from build123d import *


with BuildPart() as part:
    # Sketch1 → Revolve1 (revolve)
    with BuildSketch(Plane.XY):
        with BuildLine():
            Line((0, 8), (4.7, 8))
            ThreePointArc((4.7, 8), (4.912132034, 7.912132034), (5, 7.7))
            Line((5, 7.7), (5, 3))
            Line((5, 3), (3.5, 2))
            Line((3.5, 2), (3.5, 1.5))
            Line((3.5, 1.5), (5, 0.5))
            Line((5, 0.5), (4.711324865, 0))
            Line((4.711324865, 0), (0, 0))
            Line((0, 0), (0, 8))
        make_face()
    revolve(axis=Axis((0, 0, 0), (0, 1, 0)))

    # Sketch2 → Cut-Revolve1 (revolve, cut)
    with BuildSketch(Plane.XY):
        Polygon((0, 8), (2, 8), (2, 5), (3, 5), (3, 1), (4.711324865, 0), (0, 0), align=None)
    revolve(axis=Axis((0, 0, 0), (0, 1, 0)), mode=Mode.SUBTRACT)


solid = part.part
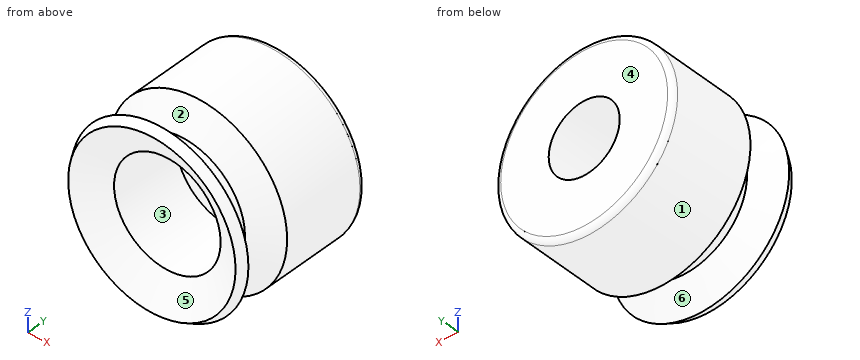
Geometry check sheet. Reference: the model listing, model coordinates, mm. Face numbers are marked on the shaded views. A direction names the side the tool comes from. Give positions to 0.01 mm unless a question says otherwise; leave off trailing zeros. Loops run counter-clockwise (first coordinate to the right, second up) from the corner with the lowest first, then second, coordinate; pieces in that order, holes last. Notation, with made-up numbers: M 24,78 L 63,78 A27 ccw 63,106 Z; hole C -18,-16 d11. An arc over 180 degrees is marked long. Write each question's results on one line, items separated by ' | '.
1) Thickness scan on line 1 (Z direction, x = 0, y = 6.8); line 2 (X direction, y = 3.5, z = 0). Record the ranges inside material, lowest first.
Answers follow:
line 1: -5 to -2, 2 to 5 | line 2: -5 to -3, 3 to 5
2) Section check A-A, the plane x = 0. Record the boundary of the cut face in (y, z), plus the area to 3 significant figures.
Answers follow:
outline: M 0,-4.71 L 0.5,-5 L 1.5,-3.5 L 2,-3.5 L 3,-5 L 7.7,-5 A0.3 ccw 8,-4.7 L 8,-2 L 5,-2 L 5,-3 L 1,-3 Z; M 0,4.71 L 1,3 L 5,3 L 5,2 L 8,2 L 8,4.7 A0.3 ccw 7.7,5 L 3,5 L 2,3.5 L 1.5,3.5 L 0.5,5 Z | area: 31.6 mm2
3) Section check C-C, the plane y = 6.5. Record the boundary of the cut face in (x, z).
Answers follow:
outline: C 0,0 d10; hole C 0,0 d4
4) Gauge pin test, flat ends, axial feed: pin 1 (2 mm diameter, centred on x = 2.5, z = 1.5, fed in from -Y); pin 2 (1 mm diameter, centred on x = 3.5, y = 3, fed in from -Z); pin 3 (3 mm diameter, centred on x = 2, y = 3, fed in from -Z). Record the tip position at first contact, or that the pin passes through.
Answers follow:
pin 1: y = 0.47 | pin 2: z = -4 | pin 3: z = -4.97
5) Section check B-B, the plane z = 0. Record the boundary of the cut face in (x, y).
Answers follow:
outline: M -5,0.5 L -4.71,0 L -3,1 L -3,5 L -2,5 L -2,8 L -4.7,8 A0.3 ccw -5,7.7 L -5,3 L -3.5,2 L -3.5,1.5 Z; M 2,5 L 3,5 L 3,1 L 4.71,0 L 5,0.5 L 3.5,1.5 L 3.5,2 L 5,3 L 5,7.7 A0.3 ccw 4.7,8 L 2,8 Z
6) Tool access check on the marked faces 1, 2 and 3. Record the directions out of +Z, -Z, +X, -X, +Y, -Y that give a thin tool (end or side, any length) a straight path to the whole face; none if there is none.
Answers follow:
face 1: +Y, -Y | face 2: none | face 3: -Y
7) Release check for a two-part mould opening along Z. For the marked faces 4, 5 and 6 record: +Z half, -Z half, draft (parallel to the pull), parting line (faces both ways), or undercut.
Answers follow:
face 4: draft | face 5: undercut | face 6: parting line
8) Section check D-D, the plane y = 3.25. Record the boundary of the cut face in (x, z).
Answers follow:
outline: C 0,0 d10; hole C 0,0 d6
